```python
from build123d import *

# Parameters (mm, degrees)
CHAMFER1_SIZE  = 1
CHAMFER1_SIZE2 = 0.577350269


with BuildPart() as part:
    # Sketch1 → Revolve1 (revolve)
    with BuildSketch(Plane.XY):
        Polygon((0, 0), (0, 6), (2, 6), (2, 4), (7.7, 4), (8, 3), (11, 3), (11.3, 4), (14.5, 4), (14.5, 0), align=None)
    revolve(axis=Axis((14.5, 0, 0), (-1, 0, 0)))

    # Chamfer1
    chamfer1_edges = [part.edges().sort_by_distance(p)[0] for p in [
        (14.5, -4, 0),
    ]]
    chamfer1_side = [part.faces().sort_by_distance(p)[0] for p in [
        (12.9, -4, 0),
    ]]
    chamfer(chamfer1_edges, length=CHAMFER1_SIZE, length2=CHAMFER1_SIZE2, reference=chamfer1_side[0])


solid = part.part
```
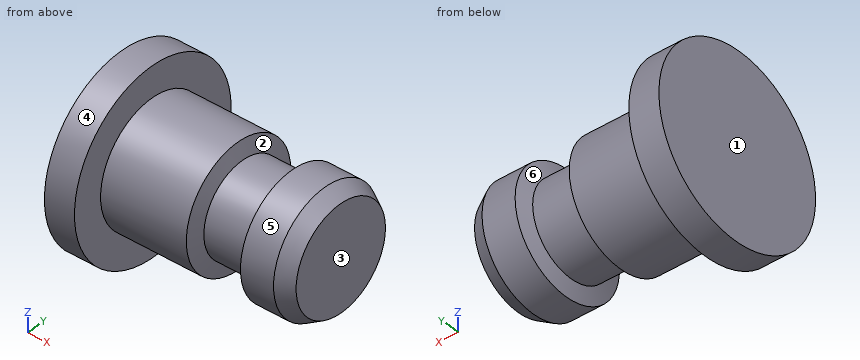
Here's how the part is built. I have some questions about the finished solid (model axes, mm). Face numbers are marked on the shaded views. A direction names the side the tool comes from. Coordinates: 2 decimals unless noted, no trailing zeros. Loops run counter-clockwise (first coordinate to the right, second up) from the corner with the lowest first, then second, coordinate; pieces in that order, holes last. Notation, with made-up numbers: M -25.5,30.5 L 26.5,30.5 A12 ccw 26.5,48.5 Z; hole C -32.75,63 d9. An arc over 180 degrees is marked long. One line per item, written item: value.
1. Please list where these lines run through material, in increasing order: probe 1 along X at (y, z) = (-4, -3.5); probe 2 along X at (y, z) = (-3.5, 1); probe 3 along Z at (x, y) = (10, 0).
Geometry says:
probe 1: x = 0 to 2
probe 2: x = 0 to 7.81, 11.19 to 14.12
probe 3: z = -3 to 3
2. Imagine slicing it at A-A (z = 0). List the corners of the cut face in (x, y) for me, and give its area (3 significant figures).
Geometry says:
outline: M 0,-6 L 2,-6 L 2,-4 L 7.7,-4 L 8,-3 L 11,-3 L 11.3,-4 L 13.5,-4 L 14.5,-3.42 L 14.5,3.42 L 13.5,4 L 11.3,4 L 11,3 L 8,3 L 7.7,4 L 2,4 L 2,6 L 0,6 Z
area: 117 mm2
3. On a 3-axis mill with a long thin cutter (end or side, diameter ignored), from which of +Z, -Z, +X, -X, +Y, -Y can I reach the whole of each face in a straight line? I mean the marked faces 4, 5 and 6. Say none if no direction works.
Geometry says:
face 4: +X, -X
face 5: +X
face 6: none
4. Imagine slicing it at C-C (x = 9.25). List the corners of the cut face in (y, z) for me, and give its area (3 significant figures).
Geometry says:
outline: C 0,0 d6
area: 28.3 mm2
5. Will these pins go through, and if not, where does the flat tip stop? pin 1 Ø5 at (x, z) = (4, 2.5) entering from -Y; pin 2 Ø4 at (x, y) = (7, 4) entering from -Z; pin 3 Ø1.5 at (x, z) = (6.5, -1) entering from +Y.
Geometry says:
pin 1: stops at y = -5.92
pin 2: stops at z = -3.46
pin 3: stops at y = 3.99
6. Thinking about a two-plate mould opening in X: for the marked faces 1, 2 and 3, which applies, +X half, -X half, draft (parallel to the pull), parting line (faces both ways), or undercut?
Geometry says:
face 1: -X half
face 2: undercut
face 3: +X half
7. Imagine slicing it at D-D (x = 5.25). List the corners of the cut face in (y, z) for me.
Geometry says:
outline: C 0,0 d8
